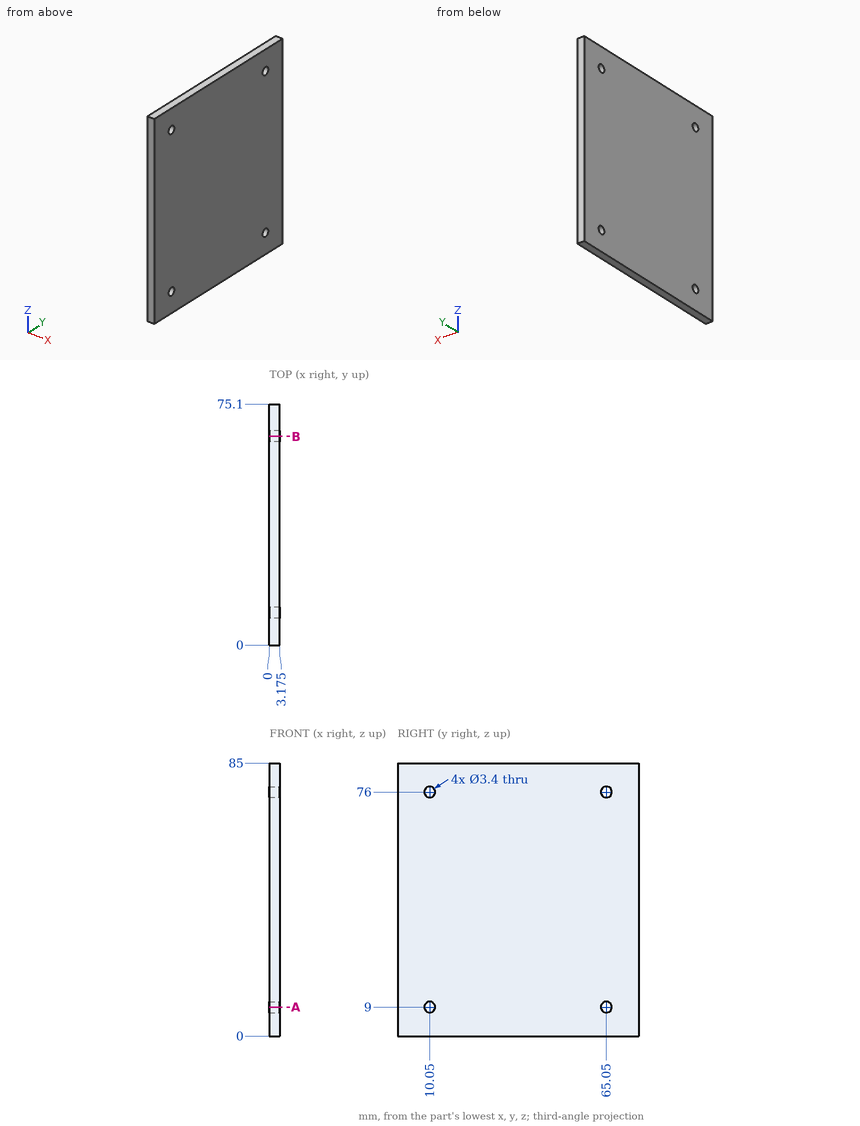
Print and shaded views of the part. All mm, measured from the part's lowest x, y and z. Coordinates: 2 decimals unless noted, no trailing zeros. Order: outer loops, then holes, each group sorted by start corner. A loop starts at its lowest first (then second) coordinate and runs counter-clockwise, first axis right, second up. Notation, with made-up numbers: (-34, 7.25) -> (-24, 7.25) arc R21 cw to (-24, 14.25) -> close; hole circle Ø8 at (74.25, 3). An arc over 180 degrees is marked (long way). Answer as a JSON object with one key per item and string values. Group by question number.
1) Drill centre lines: L1, parallel to Y at x = 1.4, z = 76; L2, parallel to Z at x = 0.6, y = 65.05; L3, parallel to Y at x = 0.4, z = 75. Where is each one in solid material? Low to high.
2) Cut at B-B, the plane y = 65.05. Write the cut outline in (x, z) (3 decimals).
3) Cut at A-A, the plane z = 9. Write the cut outline in (x, y) (3 decimals), then the cut area to 3 significant figures.
4) Flat gauge pins, fed straight in: pin 1 (1.5 mm diameter, centred on y = 21.5, z = 9, fed in from -X); pin 2 (2.5 mm diameter, centred on y = 65.05, z = 9, fed in from -X). Where does each tip first touch, or does it go through?
Check values:
{
 "1": {"L1": "y = 0 to 8.35, 11.75 to 63.35, 66.75 to 75.1", "L2": "z = 0 to 7.3, 10.7 to 74.3, 77.7 to 85", "L3": "y = 0 to 8.68, 11.42 to 63.68, 66.42 to 75.1"},
 "2": {"outline": "(0, 0) -> (3.175, 0) -> (3.175, 7.3) -> (0, 7.3) -> close; (0, 10.7) -> (3.175, 10.7) -> (3.175, 74.3) -> (0, 74.3) -> close; (0, 77.7) -> (3.175, 77.7) -> (3.175, 85) -> (0, 85) -> close"},
 "3": {"outline": "(0, 0) -> (3.175, 0) -> (3.175, 8.35) -> (0, 8.35) -> close; (0, 11.75) -> (3.175, 11.75) -> (3.175, 63.35) -> (0, 63.35) -> close; (0, 66.75) -> (3.175, 66.75) -> (3.175, 75.1) -> (0, 75.1) -> close", "area": "217 mm²"},
 "4": {"pin 1": "stops at x = 0", "pin 2": "passes through"}
}
